For this review, take the finished solid that the model builds, in its own axes (mm). Face numbers are marked on the shaded views. A direction names the side the tool comes from. Coordinates: 2 decimals unless noted, no trailing zeros. Write each loop counter-clockwise with the first axis right and the second up, starting at its lowest first coordinate (ties: lowest second). Pieces come first, ordered by that corner, then holes. Notation, with made-up numbers: (-0.5, 18.5) - (23.5, 18.5) arc R28 ccw to (23.5, 43.5) - close; hole circle Ø8 at (83, 76). An arc over 180 degrees is marked (long way). Write each question's results on one line, items separated by ' | '.
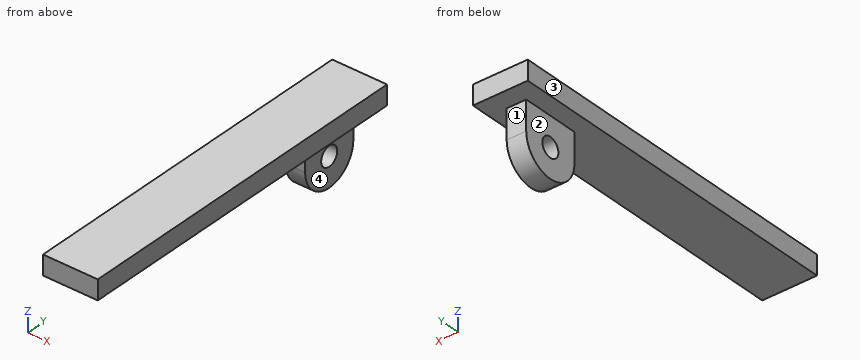
from build123d import *

# Parameters (mm, degrees)
SKETCH1_W           = 28
SKETCH1_H           = 10
BOSS_EXTRUDE1_DEPTH = 270
SKETCH2_W           = 10
SKETCH2_H           = 30
BOSS_EXTRUDE2_DEPTH = 30
SKETCH3_R           = 5
CUT_EXTRUDE1_DEPTH  = 30
SKETCH4_W           = 28
SKETCH4_H           = 90
CUT_EXTRUDE2_DEPTH  = 10


with BuildPart() as part:
    # Sketch1 → Boss-Extrude1 (new body)
    with BuildSketch(Plane(origin=(0, 0, 0), x_dir=(1, 0, 0), z_dir=(0, 1, 0))):
        Rectangle(SKETCH1_W, SKETCH1_H)
    extrude(amount=BOSS_EXTRUDE1_DEPTH)

    # Sketch2 → Boss-Extrude2 (add)
    with BuildSketch(Plane(origin=(0, 0, -5), x_dir=(-1, 0, 0), z_dir=(0, 0, -1))):
        with Locations((0, 155)):
            Rectangle(SKETCH2_W, SKETCH2_H)
    extrude(amount=BOSS_EXTRUDE2_DEPTH)

    # Sketch3 → Cut-Extrude1 (cut)
    with BuildSketch(Plane.ZY.offset(5)):
        with Locations((-20, 155)):
            Circle(SKETCH3_R)
        with BuildLine():
            Line((-20, 140), (-48.501597926, 140))
            Line((-48.501597926, 140), (-48.501597926, 172.313488336))
            Line((-48.501597926, 172.313488336), (-20, 170))
            ThreePointArc((-20, 170), (-35, 155), (-20, 140))
        make_face()
    extrude(amount=-CUT_EXTRUDE1_DEPTH, mode=Mode.SUBTRACT)

    # Sketch4 → Cut-Extrude2 (cut)
    with BuildSketch(Plane(origin=(0, 0, -5), x_dir=(-1, 0, 0), z_dir=(0, 0, -1))):
        with Locations((0, 225)):
            Rectangle(SKETCH4_W, SKETCH4_H)
    extrude(amount=-CUT_EXTRUDE2_DEPTH, mode=Mode.SUBTRACT)


solid = part.part
Q1. Take a section at D-D on y = 72. State the section outline as (x, z) points, plus the area to 3 significant figures.
Results found:
outline: (-14, -5) - (14, -5) - (14, 5) - (-14, 5) - close | area: 280 mm2
Q2. Wall thickness on line 1 along Y through (x, z) = (2, -20); line 2 along Z through (x, y) = (0.25, 98); line 3 along Y through (x, z) = (0.75, -6): over which ranges is each line inside the solid? List them lowest first. Write a range as from..to.
Results found:
line 1: 140..150, 160..170 | line 2: -5..5 | line 3: 140..170
Q3. For pin 1 (4 mm diameter, centred on x = 4, y = 31.5, fed in from -Z); pin 2 (6 mm diameter, centred on y = 155, z = -20, fed in from -X); pin 3 (4 mm diameter, centred on x = 5.5, z = -13.5, fed in from -Y); pin 4 (9 mm diameter, centred on y = 160.5, z = -13, fed in from -X), all flat-tipped, find the tip position at first contact; note any pin that passes through.
Results found:
pin 1: z = -5 | pin 2: through | pin 3: y = 140 | pin 4: x = -5
Q4. For the marked faces 1, 2, 3 and 4, list the 3-axis set-ups (+Z, -Z, +X, -X, +Y, -Y) from which the entire face can be reached by the end or side of a thin tool; tool diameter is ignored.
Results found:
face 1: -Z, +X, -X, +Y | face 2: -Z, -X, +Y, -Y | face 3: +Z, -Z, -X, +Y, -Y | face 4: -Z, +X, +Y, -Y
Q5. Take a section at A-A on y = 155. State the section outline as (x, z) points, plus the area to 3 significant figures.
Results found:
outline: (-14, -5) - (-5, -5) - (-5, -15) - (5, -15) - (5, -5) - (14, -5) - (14, 5) - (-14, 5) - close; (-5, -35) - (5, -35) - (5, -25) - (-5, -25) - close | area: 480 mm2
Q6. Take a section at B-B on x = 0.5. State the section outline as (y, z) points.
Results found:
outline: (0, -5) - (140, -5) - (140, -20) arc R15 ccw to (170, -20) - (170, -5) - (180, -5) - (180, 5) - (0, 5) - close; hole circle Ø10 at (155, -20)
Q7. Take a section at C-C on z = -7.5. State the section outline as (x, y) points, plus the area to 3 significant figures.
Results found:
outline: (-5, 140) - (5, 140) - (5, 170) - (-5, 170) - close | area: 300 mm2
